```python
from build123d import *

# Parameters (mm, degrees)
SKETCH2_W          = 3
SKETCH2_H          = 3.5
SKETCH2_H_2        = 1.5
SKETCH2_W_2        = 9
SKETCH2_6_W        = 30
SKETCH2_6_H        = 3
SKETCH3_R          = 1.5
CUT_EXTRUDE1_DEPTH = 3.5
SKETCH4_R          = 1.75
CUT_EXTRUDE2_DEPTH = 104.464679964


with BuildPart() as part:
    # Sketch2 → Revolve2 (revolve)
    with BuildSketch(Plane.XY, mode=Mode.PRIVATE) as revolve2_sk:
        Polygon((0, 14.5), (37.5, 14.5), (37.5, 29), (0, 29), (0, 19.5), (0, 16), align=None)
        Polygon((37.5, 29), (37.5, 14.5), (60, 14.5), (60, 15.5), (60, 21.5), (60, 27.5), (60, 33), (37.5, 33), align=None)
        with Locations((-1.5, 17.75)):
            Rectangle(SKETCH2_W, SKETCH2_H)
        with Locations((-1.5, 15.25)):
            Rectangle(SKETCH2_W, SKETCH2_H_2)
        with Locations((-7.5, 15.25)):
            Rectangle(SKETCH2_W_2, SKETCH2_H_2)
    revolve(revolve2_sk.sketch.rotate(Axis((-31.266871865, 14.5, 0), (1, 0, 0)), 90), axis=Axis((-31.266871865, 14.5, 0), (1, 0, 0)))

    # Sketch2<6> → Revolve3 (revolve)
    with BuildSketch(Plane.XY, mode=Mode.PRIVATE) as revolve3_sk:
        Polygon((60, 27.5), (60, 21.5), (66.3, 21.5), (66.3, 24.5), (66.3, 27.5), align=None)
        with Locations((81.3, 23)):
            Rectangle(SKETCH2_6_W, SKETCH2_6_H)
    revolve(revolve3_sk.sketch.rotate(Axis((60, 21.5, 0), (1, 0, 0)), 90), axis=Axis((60, 21.5, 0), (1, 0, 0)))

    # Sketch3 → Cut-Extrude1 (cut)
    with BuildSketch(Plane(origin=(60, 0, 0), x_dir=(0, 0, -1), z_dir=(1, 0, 0))):
        with Locations((-15.5, 14.5)):
            Circle(SKETCH3_R)
        with Locations((-7.75, 27.923393759)):
            Circle(SKETCH3_R)
        with Locations((7.75, 27.923393759)):
            Circle(SKETCH3_R)
        with Locations((15.5, 14.5)):
            Circle(SKETCH3_R)
        with Locations((7.75, 1.076606241)):
            Circle(SKETCH3_R)
        with Locations((-7.75, 1.076606241)):
            Circle(SKETCH3_R)
    extrude(amount=-CUT_EXTRUDE1_DEPTH, mode=Mode.SUBTRACT)

    # Sketch4 → Cut-Extrude2 (cut, through all)
    with BuildSketch(Plane(origin=(0, 0, 0), x_dir=(1, 0, 0), z_dir=(0, 1, 0))):
        with Locations(Location((87.8, 0, 0), (0, 0, 90))):
            Circle(SKETCH4_R)
    extrude(amount=CUT_EXTRUDE2_DEPTH, mode=Mode.SUBTRACT)


solid = part.part
```
Here's how the part is built. I have some questions about the finished solid (model axes, mm). A direction names the side the tool comes from. Round coordinates to 2 decimals unless told otherwise and drop trailing zeros. Write each loop counter-clockwise with the first axis right and the second up, starting at its lowest first coordinate (ties: lowest second). Pieces come first, ordered by that corner, then holes. Notation, with made-up numbers: M 2.5,37 L 35.5,37 A33 ccw 35.5,68 Z; hole C 48.5,87 d6. An arc over 180 degrees is marked long. Answer as CSV lines item,"result". Start each with the question number.
1. Suppose I cut it at A-A on x = 58.5. Write out the boundary of the cut face in (y, z).
2. I'm going to push flat-ended pins straight in: pin 1 Ø5 at (y, z) = (27.92, 7.75) entering from -X; pin 2 Ø12 at (y, z) = (5, 6) entering from +X; pin 3 Ø1.8 at (y, z) = (14.5, 15.5) entering from -X. Where does each tip first touch, or does it pass through?
3. On a 3-axis mill with a long thin cutter (end or side, diameter ignored), from which of +Z, -Z, +X, -X, +Y, -Y can I reach the whole of each face in a straight line? I mean faces 4 (the flat face through (-3, 16, -1)), 5 (the cylindrical face through (58.27, 1.14, 9.25)), 6 (the flat face through (96.3, 21, 0)). Say none if no direction works.
4. Suppose I cut it at D-D on y = 21.5. Write out the boundary of the cut face in (x, z).
5. I need wall thicknesses on probe 1 along X at (y, z) = (24, 9); probe 2 along X at (y, z) = (0.5, -12); probe 3 along Y at (x, z) = (57, 15). Which ranges of each line are inside material? Lowest first, please.
6. Suppose I cut it at B-B on y = 14.5. Write out the boundary of the cut face in (x, z), then the cut area to 3 significant figures.
7. Thinking about a two-plate mould opening in Y: for faces 1 (the flat face through (-12, 14, 0)), 2 (the flat face through (56.5, 15, 16)), 3 (the cylindrical face through (63.11, 15.55, -0.78)), which applies, released by +Y, released by -Y, zero draft, split by the parting line, or undercut?
8. Suppose I cut it at C-C on z = -7.75. Write out the boundary of the cut face in (x, y).
Check result:
1,outline,"C 14.5,0 d37; hole C 1.08,-7.75 d3; hole C 1.08,7.75 d3; hole C 14.5,-15.5 d3; hole C 14.5,15.5 d3; hole C 27.92,-7.75 d3; hole C 27.92,7.75 d3"
2,pin 1,"stops at x = 0"
2,pin 2,"stops at x = 60"
2,pin 3,"stops at x = 37.5"
3,face 4,"-X"
3,face 5,"+X"
3,face 6,"+Z, -Z, +X, +Y, -Y"
4,outline,"M 0,-12.7 L 37.5,-12.7 L 37.5,-17.12 L 60,-17.12 L 60,-6 L 66.3,-6 L 66.3,-3 L 96.3,-3 L 96.3,3 L 66.3,3 L 66.3,6 L 60,6 L 60,17.12 L 37.5,17.12 L 37.5,12.7 L 0,12.7 Z; hole C 87.8,0 d3.5"
5,probe 1,"x = 0 to 60"
5,probe 2,"x = 37.5 to 60"
5,probe 3,"y = 3.67 to 13.09, 15.91 to 25.33"
6,outline,"M -12,-1.5 L -3,-1.5 L -3,-5 L 0,-5 L 0,-14.5 L 37.5,-14.5 L 37.5,-18.5 L 60,-18.5 L 60,-17 L 56.5,-17 L 56.5,-14 L 60,-14 L 60,14 L 56.5,14 L 56.5,17 L 60,17 L 60,18.5 L 37.5,18.5 L 37.5,14.5 L 0,14.5 L 0,5 L -3,5 L -3,1.5 L -12,1.5 Z"
6,area,"1,960 mm2"
7,face 1,"zero draft"
7,face 2,"undercut"
7,face 3,"split by the parting line"
8,outline,"M 0,2.24 L 37.5,2.24 L 37.5,-2.3 L 60,-2.3 L 60,-0.42 L 56.5,-0.42 L 56.5,2.58 L 60,2.58 L 60,26.42 L 56.5,26.42 L 56.5,29.42 L 60,29.42 L 60,31.3 L 37.5,31.3 L 37.5,26.76 L 0,26.76 Z"
